Could you check a few things on this model? Use its own coordinates, in mm. A direction names the side the tool comes from. Give positions to 0.01 mm unless a question says otherwise; leave off trailing zeros. Loops run counter-clockwise (first coordinate to the right, second up) from the corner with the lowest first, then second, coordinate; pieces in that order, holes last. Notation, with made-up numbers: M -30.5,52.25 L 0.5,52.25 A22 cw 0.5,81.25 Z; hole C 12.25,-27 d5. An arc over 180 degrees is marked long. Write each question's results on one line, items separated by ' | '. Start each with the question number.
from build123d import *

# Parameters (mm, degrees)
SKETCH1_R           = 25.4
BOSS_EXTRUDE5_DEPTH = 12.7
SKETCH4_9_R         = 49.587536422
CUT_EXTRUDE9_DEPTH  = 12.7
SKETCH4_10_R        = 3.175
CUT_EXTRUDE10_DEPTH = 6.35


with BuildPart() as part:
    # Sketch1 → Boss-Extrude5 (new body)
    with BuildSketch(Plane(origin=(0, 0, 0), x_dir=(1, 0, 0), z_dir=(0, 1, 0))):
        with BuildLine():
            Line((63.881, 0), (63.881, -127))
            ThreePointArc((63.881, -127), (0, -190.881), (-63.881, -127))
            Line((-63.881, -127), (-63.881, 0))
            ThreePointArc((-63.881, 0), (-53.533587031, 34.855949573), (-25.843485852, 58.42))
            Line((-25.843485852, 58.42), (0, 58.42))
            Line((0, 58.42), (25.843485852, 58.42))
            ThreePointArc((25.843485852, 58.42), (39.052759066, 50.553577226), (50.000033281, 39.759009455))
            Line((50.000033281, 39.759009455), (68.760605235, 48.322238074))
            Line((68.760605235, 48.322238074), (74.445380321, 35.867866389))
            Line((74.445380321, 35.867866389), (43.162005956, 21.588627605))
            ThreePointArc((43.162005956, 21.588627605), (-43.902763298, -20.039335689), (44.587930732, 18.464669861))
            Line((44.587930732, 18.464669861), (75.871305097, 32.743908644))
            Line((75.871305097, 32.743908644), (81.556080183, 20.289536959))
            Line((81.556080183, 20.289536959), (62.795508229, 11.726308341))
            ThreePointArc((62.795508229, 11.726308341), (63.609048186, 5.888221287), (63.881, 0))
        make_face()
        with Locations((0, -127)):
            Circle(SKETCH1_R, mode=Mode.SUBTRACT)
    extrude(amount=BOSS_EXTRUDE5_DEPTH)

    # Sketch4_9 → Cut-Extrude9 (cut)
    with BuildSketch(Plane(origin=(0, 0, 0), x_dir=(1, 0, 0), z_dir=(0, 1, 0))):
        Circle(SKETCH4_9_R)
    extrude(amount=CUT_EXTRUDE9_DEPTH, mode=Mode.SUBTRACT)

    # Sketch4_10 → Cut-Extrude10 (cut)
    with BuildSketch(Plane(origin=(0, 0, 0), x_dir=(1, 0, 0), z_dir=(0, 1, 0))):
        with Locations((0, -171.45)):
            Circle(SKETCH4_10_R)
        with Locations((-44.45, -127)):
            Circle(SKETCH4_10_R)
        with Locations((44.45, -127)):
            Circle(SKETCH4_10_R)
        with Locations((0, -82.55)):
            Circle(SKETCH4_10_R)
        with Locations((-44.45, -41.311332975)):
            Circle(SKETCH4_10_R)
        with Locations((44.45, -45.306446958)):
            Circle(SKETCH4_10_R)
    extrude(amount=CUT_EXTRUDE10_DEPTH, mode=Mode.SUBTRACT)


solid = part.part
1) If we section it at A-A on x = 0: Write out the boundary of the cut face in (y, z) (3 decimals), plus the area to 3 significant figures.
2) Please list where these lines run through material, in increasing order: line 1 (X direction, y = 1.5, z = 127) (3 decimals); line 2 (Z direction, x = 44.45, y = 3.5) (3 decimals); line 3 (Z direction, x = -13, y = 6.75). Write a range as from..to.
3) If we section it at D-D on z = 82.55: Write out the boundary of the cut face in (x, y) (3 decimals).
4) Thinking about a two-plate mould opening in Z: for faces 5 (the face through (44, 6.35, 45)), 6 (the face through (0, 6, -58.42)), 7 (the face through (1.405, 6.261, 190.866)), which applies, pulls with the +Z half, pulls with the -Z half, needs draft (parallel to the pull), parting line crosses it, or undercut?
5) If we section it at B-B on x = 59: Write out the boundary of the cut face in (y, z).
6) Which directions (+Z, -Z, +X, -X, +Y, -Y) give clear straight access to the entire face, cutting with the end or side of a thin tool? Please do faces 1 (the face through (63.881, 6, 63)), 2 (the face through (59.62, 6.26, -29.1)), 3 (the face through (0, 6.35, 171)), 4 (the face through (59.25, 6.26, -43.98)).
7) If we section it at C-C on y = 3: State how many separate pieces and enclosed holes the cut face has, plus the area to 3 significant figures.
8) I'm going to push flat-ended pins straight in: P1, Ø1.9, axis at x = -45, z = 127, coming from the -Y side; P2, Ø3, axis at y = 10, z = -24.5, coming from the -X side; P3, Ø1, axis at x = 42.5, y = 3, coming from the +Z side. Where does each tip first touch, or does it pass through?
Calculated:
1) outline: M 0,-58.42 L 12.7,-58.42 L 12.7,-49.588 L 0,-49.588 Z; M 0,49.588 L 12.7,49.588 L 12.7,101.6 L 0,101.6 L 0,85.725 L 6.35,85.725 L 6.35,79.375 L 0,79.375 Z; M 0,152.4 L 12.7,152.4 L 12.7,190.881 L 0,190.881 L 0,174.625 L 6.35,174.625 L 6.35,168.275 L 0,168.275 Z | area: 1,180 mm2
2) line 1: x = -63.881..-47.625, -41.275..-25.4, 25.4..41.275, 47.625..63.881 | line 2: z = -45.88..-22.177, 21.98..42.131, 48.481..123.825, 130.175..172.88 | line 3: z = -58.42..-47.85, 47.85..105.18, 148.82..189.54
3) outline: M -63.881,0 L -3.175,0 L -3.175,6.35 L 3.175,6.35 L 3.175,0 L 63.881,0 L 63.881,12.7 L -63.881,12.7 Z
4) face 5: undercut | face 6: pulls with the -Z half | face 7: pulls with the +Z half
5) outline: M 0,-43.87 L 12.7,-43.87 L 12.7,-28.82 L 0,-28.82 Z; M 0,-25.04 L 12.7,-25.04 L 12.7,151.49 L 0,151.49 Z
6) face 1: +Z, +X, +Y, -Y | face 2: +Y, -Y | face 3: -Y | face 4: -Z, +Y, -Y
7) separate pieces: 1 | enclosed holes: 7 | area: 19,400 mm2
8) P1: stops at y = 6.35 | P2: stops at x = -59.6 | P3: stops at z = 175.13
